Geometry: final body of the model. Coordinates: model frame, mm. A direction names the side the tool comes from. Give positions to 0.01 mm unless a question says otherwise; leave off trailing zeros. Write each loop counter-clockwise with the first axis right and the second up, starting at its lowest first coordinate (ties: lowest second). Pieces come first, ordered by that corner, then holes. Notation, with made-up numbers: (-22.5, 88) -> (25.5, 88) arc R29 cw to (25.5, 108) -> close; hole circle Ø2 at (-26.5, 14.5). An arc over 180 degrees is marked (long way). Use CSV: the item, a comma, the result in double quotes. Start each with the question number.
1) Section D-D (x = 474). Output: boundary loops of the cut face in (y, z), plus the area to 3 significant figures.
2) Section B-B (x = 748). Output: boundary loops of the cut face in (y, z), plus the area to 3 significant figures.
3) Section C-C (y = 201.5). Output: boundary loops of the cut face in (x, z).
4) Section A-A (z = -274.5). Output: boundary loops of the cut face in (x, y).
5) Set-up query: faces 1 (the face through (1144, 740, -560)), 2 (the face through (660, 45, -934)), 3 (the face through (1320, 755, -556)), 4 (the face through (660, 45, -299)). Return all of +Z, -Z, +X, -X, +Y, -Y with unobstructed straight access to the full face (end or side cutting, diameter ignored); none if empty.
6) Material intervals for line 1 (Z direction, x = 300.5, y = 453.5); line 2 (Z direction, x = 669, y = 701.5); line 3 (X direction, y = 364, z = -868), sorted ascending. Write a range as [from, to].
7) Contact query for flat-ended pins moving along their axis: P1, Ø1, axis at x = 1123, y = 335.5, coming from the -Z side; P2, Ø24, axis at y = 751.5, z = -415, coming from the -X side; P3, Ø9, axis at x = 677.5, z = -384.5, coming from the -Y side. Output: stop coordinate, or through.
8) Draft query along Y for faces 5 (the face through (672, 770, -597)), 6 (the face through (666, 2, -51)), 7 (the face through (60, 755, -671)). Return one class per face: pulls with the +Y half, pulls with the -Y half, needs draft (parallel to the pull), parting line crosses it, or undercut.
```python
from build123d import *

# Parameters (mm, degrees)
F1_DEPTH      = 1350
F2_R          = 50
F3_W          = 30
F3_H          = 30
F4_DEPTH      = 865
F5_W          = 740
F5_H          = 30
F6_DEPTH      = 630
F6_DEPTH_BACK = 30
F7_W          = 30
F7_H          = 30
F8_DEPTH      = 600
F9_W          = 30
F9_H          = 30
F10_DEPTH     = 680


with BuildPart() as f1:
    # F0 (on Right) → F1 (new body)
    with BuildSketch(Plane.YZ):
        Polygon((2, 0), (0, 0), (0, -130), (800, -130), (800, 0), (798, 0), (798, -100), (2, -100), align=None)
    extrude(amount=F1_DEPTH)

    # F2
    f2_edges = [f1.edges().sort_by_distance(p)[0] for p in [
        (1350, 1, 0),
        (1350, 799, 0),
        (0, 799, 0),
        (0, 1, 0),
    ]]
    fillet(f2_edges, radius=F2_R)

    # F3 (on face) → F4 (join)
    with BuildSketch(Plane(origin=(0, 0, -130), x_dir=(1, 0, 0), z_dir=(0, 0, -1))):
        with Locations((45, -45)):
            Rectangle(F3_W, F3_H)
        with Locations((1305, -45)):
            Rectangle(F3_W, F3_H)
        with Locations((1305, -755)):
            Rectangle(F3_W, F3_H)
        with Locations((45, -755)):
            Rectangle(F3_W, F3_H)
        with Locations((675, -45)):
            Rectangle(F3_W, F3_H)
        with Locations((675, -755)):
            Rectangle(F3_W, F3_H)
    extrude(amount=F4_DEPTH)

    # F5 (on face) → F6 (join, two sides)
    with BuildSketch(Plane.YZ.offset(60)) as f6_sk:
        with Locations((400, -860)):
            Rectangle(F5_W, F5_H)
        with Locations((400, -487.5)):
            Rectangle(F5_W, F5_H)
    extrude(amount=F6_DEPTH)
    extrude(f6_sk.sketch, amount=-F6_DEPTH_BACK)

    # F7 (on face) → F8 (join, through all)
    with BuildSketch(Plane.YZ.offset(690)):
        with Locations((45, -562.5)):
            Rectangle(F7_W, F7_H)
        with Locations((755, -562.5)):
            Rectangle(F7_W, F7_H)
    extrude(amount=F8_DEPTH)

    # F9 (on face) → F10 (join, through all)
    with BuildSketch(Plane.XZ.offset(-740)):
        with Locations((675, -562.5)):
            Rectangle(F9_W, F9_H)
    extrude(amount=F10_DEPTH)


solid = f1.part
```
Answers follow:
1,outline,"(0, -130) -> (800, -130) -> (800, 0) -> (798, 0) -> (798, -100) -> (2, -100) -> (2, 0) -> (0, 0) -> close; (30, -875) -> (770, -875) -> (770, -845) -> (30, -845) -> close; (30, -502.5) -> (770, -502.5) -> (770, -472.5) -> (30, -472.5) -> close"
1,area,"68,800 mm^2"
2,outline,"(0, -130) -> (800, -130) -> (800, 0) -> (798, 0) -> (798, -100) -> (2, -100) -> (2, 0) -> (0, 0) -> close; (30, -577.5) -> (60, -577.5) -> (60, -547.5) -> (30, -547.5) -> close; (740, -577.5) -> (770, -577.5) -> (770, -547.5) -> (740, -547.5) -> close"
2,area,"26,200 mm^2"
3,outline,"(0, -130) -> (1350, -130) -> (1350, -100) -> (0, -100) -> close; (30, -875) -> (690, -875) -> (690, -845) -> (30, -845) -> close; (30, -502.5) -> (690, -502.5) -> (690, -472.5) -> (30, -472.5) -> close; (660, -577.5) -> (690, -577.5) -> (690, -547.5) -> (660, -547.5) -> close"
4,outline,"(30, 30) -> (60, 30) -> (60, 60) -> (30, 60) -> close; (30, 740) -> (60, 740) -> (60, 770) -> (30, 770) -> close; (660, 30) -> (690, 30) -> (690, 60) -> (660, 60) -> close; (660, 740) -> (690, 740) -> (690, 770) -> (660, 770) -> close; (1290, 30) -> (1320, 30) -> (1320, 60) -> (1290, 60) -> close; (1290, 740) -> (1320, 740) -> (1320, 770) -> (1290, 770) -> close"
5,face 1,"-Z, +X"
5,face 2,"-Z, +Y, -Y"
5,face 3,"-Z, +X, +Y, -Y"
5,face 4,"+Y, -Y"
6,line 1,"z = [-875, -845], [-502.5, -472.5], [-130, -100]"
6,line 2,"z = [-875, -845], [-577.5, -547.5], [-502.5, -472.5], [-130, -100]"
6,line 3,"x = [30, 690]"
7,P1,"stops at z = -130"
7,P2,"stops at x = 30"
7,P3,"stops at y = 30"
8,face 5,"pulls with the +Y half"
8,face 6,"undercut"
8,face 7,"needs draft"
